Check sheet for the modelled part. Datum: model origin and axes. Units: mm. Face numbers are marked on the shaded views. Coordinates: 2 decimals unless noted, no trailing zeros. Loops run counter-clockwise (first coordinate to the right, second up) from the corner with the lowest first, then second, coordinate; pieces in that order, holes last. Notation, with made-up numbers: (39.5, 27) -> (70.5, 27) arc R20 cw to (70.5, 39) -> close; hole circle Ø1 at (-28.75, -19). An arc over 180 degrees is marked (long way). Use one line per item in the form item = value.
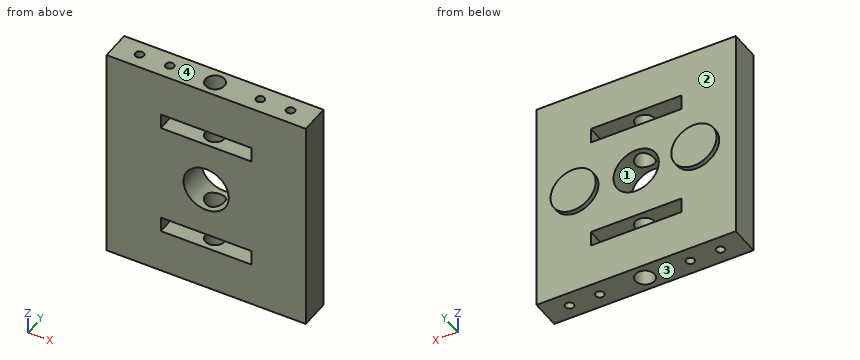
from build123d import *

# Parameters (mm, degrees)
SKETCH1_W               = 66
SKETCH1_H               = 72
BOSS_EXTRUDE1_DEPTH     = 10
SKETCH2_R               = 1.4
CUT_EXTRUDE1_DEPTH      = 10
CUT_EXTRUDE2_DEPTH      = 50.849774322
CUT_EXTRUDE2_DEPTH_BACK = 50.849774322
SKETCH3_W               = 30
SKETCH3_H               = 5
CUT_EXTRUDE3_DEPTH      = 80.831071645
CUT_EXTRUDE3_DEPTH_BACK = 80.831071645
SKETCH4_R               = 3.15
SKETCH5_R               = 7.5
BOSS_EXTRUDE2_DEPTH     = 1.5
CUT_EXTRUDE4_DEPTH      = 50.849774322
CUT_EXTRUDE4_DEPTH_BACK = 50.849774322
SKETCH6_R               = 7.5


with BuildPart() as part:
    # Sketch1 → Boss-Extrude1 (new body)
    with BuildSketch(Plane(origin=(0, 0, 0), x_dir=(1, 0, 0), z_dir=(0, 1, 0))):
        Rectangle(SKETCH1_W, SKETCH1_H)
    extrude(amount=BOSS_EXTRUDE1_DEPTH)

    # Sketch2 → Cut-Extrude1 (cut)
    with BuildSketch(Plane.XY.offset(36)):
        with Locations((-15, 5)):
            Circle(SKETCH2_R)
        with Locations((15, 5)):
            Circle(SKETCH2_R)
        with Locations((-25, 5)):
            Circle(SKETCH2_R)
        with Locations((25, 5)):
            Circle(SKETCH2_R)
    cut_extrude1 = extrude(amount=-CUT_EXTRUDE1_DEPTH, mode=Mode.SUBTRACT)

    # Mirror1: Cut-Extrude1 across plane
    add(cut_extrude1.mirror(Plane.XY), mode=Mode.SUBTRACT)

    # Sketch3 → Cut-Extrude2 (cut, two sides: drawn at the far end of the back side and taken through both)
    with BuildSketch(Plane(origin=(0, 10, 0), x_dir=(1, 0, 0), z_dir=(0, 1, 0)).offset(-CUT_EXTRUDE2_DEPTH_BACK)):
        with Locations((0, -19)):
            Rectangle(SKETCH3_W, SKETCH3_H)
        with Locations((0, 19)):
            Rectangle(SKETCH3_W, SKETCH3_H)
    extrude(amount=CUT_EXTRUDE2_DEPTH + CUT_EXTRUDE2_DEPTH_BACK, mode=Mode.SUBTRACT)

    # Sketch4 → Cut-Extrude3 (cut, two sides: drawn at the far end of the back side and taken through both)
    with BuildSketch(Plane.XY.offset(36).offset(-CUT_EXTRUDE3_DEPTH_BACK)):
        with Locations((0, 5)):
            Circle(SKETCH4_R)
    extrude(amount=CUT_EXTRUDE3_DEPTH + CUT_EXTRUDE3_DEPTH_BACK, mode=Mode.SUBTRACT)

    # Sketch5 → Boss-Extrude2 (add)
    with BuildSketch(Plane(origin=(0, 10, 0), x_dir=(1, 0, 0), z_dir=(0, 1, 0))):
        with Locations(Location((-20, 0, 0), (0, 0, 90))):
            Circle(SKETCH5_R)
        with Locations(Location((20, 0, 0), (0, 0, 90))):
            Circle(SKETCH5_R)
    extrude(amount=BOSS_EXTRUDE2_DEPTH)

    # Sketch6 → Cut-Extrude4 (cut, two sides: drawn at the far end of the back side and taken through both)
    with BuildSketch(Plane(origin=(0, 10, 0), x_dir=(1, 0, 0), z_dir=(0, 1, 0)).offset(-CUT_EXTRUDE4_DEPTH_BACK)):
        with Locations(Location((0, 0, 0), (0, 0, 270))):
            Circle(SKETCH6_R)
    extrude(amount=CUT_EXTRUDE4_DEPTH + CUT_EXTRUDE4_DEPTH_BACK, mode=Mode.SUBTRACT)


solid = part.part
(1) Section check D-D, the plane z = 0. Record the boundary of the cut face in (x, y), plus the area to 3 significant figures.
Established:
outline = (-33, 0) -> (-7.5, 0) -> (-7.5, 10) -> (-12.5, 10) -> (-12.5, 11.5) -> (-27.5, 11.5) -> (-27.5, 10) -> (-33, 10) -> close; (7.5, 0) -> (33, 0) -> (33, 10) -> (27.5, 10) -> (27.5, 11.5) -> (12.5, 11.5) -> (12.5, 10) -> (7.5, 10) -> close
area = 555 mm²
(2) Go/stop test with flat-tipped pins: P1, Ø2, axis at x = -25, y = 5, coming from the -Z side; P2, Ø1, axis at x = -8.5, z = 21.5, coming from the +Y side; P3, Ø2.5, axis at x = 15, y = 5, coming from the +Z side. Record where each tip stops, or that it passes through.
Established:
P1 = -26
P2 = 10
P3 = 26
(3) Section check A-A, the plane x = 0. Give the number of separate pieces and of enclosed holes in the cut face, plus the area to 3 significant figures.
Established:
separate_pieces = 8
enclosed_holes = 0
area = 174 mm²
(4) Section check C-C, the plane x = -11.5. Record the boundary of the cut face in (y, z).
Established:
outline = (0, -36) -> (10, -36) -> (10, -21.5) -> (0, -21.5) -> close; (0, -16.5) -> (10, -16.5) -> (10, 16.5) -> (0, 16.5) -> close; (0, 21.5) -> (10, 21.5) -> (10, 36) -> (0, 36) -> close
(5) Section check B-B, the plane y = 9. Record the boundary of the cut face in (x, z).
Established:
outline = (-33, -36) -> (33, -36) -> (33, 36) -> (-33, 36) -> close; hole (-15, -21.5) -> (15, -21.5) -> (15, -16.5) -> (-15, -16.5) -> close; hole (-15, 16.5) -> (15, 16.5) -> (15, 21.5) -> (-15, 21.5) -> close; hole circle Ø15 at (0, 0)
(6) Scan lines: line 1 along Z through (x, y) = (8.5, 1.5); line 2 along Y through (x, z) = (0, 29.5); line 3 along Z through (x, y) = (-6.5, 5.25). Record each from-to range of solid material in increasing order.
Established:
line_1 = -36 to -21.5, -16.5 to 16.5, 21.5 to 36
line_2 = 0 to 1.85, 8.15 to 10
line_3 = -36 to -21.5, -16.5 to -3.74, 3.74 to 16.5, 21.5 to 36
(7) Mould release check, pull along Z, two halves, no side actions. Record for the marked faces 1, 2, 3 and 4: +Z half, -Z half, draft (parallel to the pull), parting line (faces both ways), or undercut.
Established:
face_1 = undercut
face_2 = draft
face_3 = -Z half
face_4 = +Z half
